```python
from build123d import *

# Parameters (mm, degrees)
BOSS_EXTRUDE1_DEPTH = 3.81


with BuildPart() as part:
    # Sketch1 → Boss-Extrude1 (new body)
    with BuildSketch(Plane.XY):
        with BuildLine():
            Line((-43.434, -9.779), (-43.434, -14.224))
            Line((-43.434, -14.224), (-34.544, -14.224))
            Line((-34.544, -14.224), (-34.544, -9.779))
            Line((-34.544, -9.779), (-34.544, -8.876475723))
            ThreePointArc((-34.544, -8.876475723), (-34.231125677, -8.041724001), (-33.446660728, -7.618267365))
            Line((-33.446660728, -7.618267365), (-11.222947321, -4.568563784))
            ThreePointArc((-11.222947321, -4.568563784), (0, -3.802107076), (11.222947321, -4.568563784))
            Line((11.222947321, -4.568563784), (33.446660728, -7.618267365))
            ThreePointArc((33.446660728, -7.618267365), (34.231125677, -8.041724001), (34.544, -8.876475723))
            Line((34.544, -8.876475723), (34.544, -9.779))
            Line((34.544, -9.779), (34.544, -14.224))
            Line((34.544, -14.224), (43.434, -14.224))
            Line((43.434, -14.224), (43.434, -9.779))
            Line((43.434, -9.779), (43.434, -6.250721328))
            ThreePointArc((43.434, -6.250721328), (43.288497568, -5.660462724), (42.885330364, -5.205454612))
            ThreePointArc((42.885330364, -5.205454612), (42.48216316, -4.7504465), (42.336660728, -4.160187897))
            Line((42.336660728, -4.160187897), (42.336660728, 4.160187897))
            ThreePointArc((42.336660728, 4.160187897), (42.48216316, 4.7504465), (42.885330364, 5.205454612))
            ThreePointArc((42.885330364, 5.205454612), (43.288497568, 5.660462724), (43.434, 6.250721328))
            Line((43.434, 6.250721328), (43.434, 9.779))
            Line((43.434, 9.779), (43.434, 14.224))
            Line((43.434, 14.224), (34.544, 14.224))
            Line((34.544, 14.224), (34.544, 9.779))
            Line((34.544, 9.779), (34.544, 8.876475723))
            ThreePointArc((34.544, 8.876475723), (34.231125677, 8.041724001), (33.446660728, 7.618267365))
            Line((33.446660728, 7.618267365), (11.222947321, 4.568563784))
            ThreePointArc((11.222947321, 4.568563784), (0, 3.802107076), (-11.222947321, 4.568563784))
            Line((-11.222947321, 4.568563784), (-33.446660728, 7.618267365))
            ThreePointArc((-33.446660728, 7.618267365), (-34.231125677, 8.041724001), (-34.544, 8.876475723))
            Line((-34.544, 8.876475723), (-34.544, 9.779))
            Line((-34.544, 9.779), (-34.544, 14.224))
            Line((-34.544, 14.224), (-43.434, 14.224))
            Line((-43.434, 14.224), (-43.434, 9.779))
            Line((-43.434, 9.779), (-43.434, 6.250721328))
            ThreePointArc((-43.434, 6.250721328), (-43.288497568, 5.660462724), (-42.885330364, 5.205454612))
            ThreePointArc((-42.885330364, 5.205454612), (-42.48216316, 4.7504465), (-42.336660728, 4.160187897))
            Line((-42.336660728, 4.160187897), (-42.336660728, -4.160187897))
            ThreePointArc((-42.336660728, -4.160187897), (-42.48216316, -4.7504465), (-42.885330364, -5.205454612))
            ThreePointArc((-42.885330364, -5.205454612), (-43.288497568, -5.660462724), (-43.434, -6.250721328))
            Line((-43.434, -6.250721328), (-43.434, -9.779))
        make_face()
        with BuildLine():
            Line((-33.101339272, -3.725173331), (-15.12414212, -1.258208358))
            ThreePointArc((-15.12414212, -1.258208358), (-14.026802848, 0), (-15.12414212, 1.258208358))
            Line((-15.12414212, 1.258208358), (-33.101339272, 3.725173331))
            ThreePointArc((-33.101339272, 3.725173331), (-34.108751722, 3.42409065), (-34.544, 2.466964972))
            Line((-34.544, 2.466964972), (-34.544, -2.466964972))
            ThreePointArc((-34.544, -2.466964972), (-34.108751722, -3.42409065), (-33.101339272, -3.725173331))
        make_face(mode=Mode.SUBTRACT)
        with BuildLine():
            Line((34.544, -2.466964972), (34.544, 2.466964972))
            ThreePointArc((34.544, 2.466964972), (34.108751722, 3.42409065), (33.101339272, 3.725173331))
            Line((33.101339272, 3.725173331), (15.12414212, 1.258208358))
            ThreePointArc((15.12414212, 1.258208358), (14.026802848, 0), (15.12414212, -1.258208358))
            Line((15.12414212, -1.258208358), (33.101339272, -3.725173331))
            ThreePointArc((33.101339272, -3.725173331), (34.108751722, -3.42409065), (34.544, -2.466964972))
        make_face(mode=Mode.SUBTRACT)
    extrude(amount=BOSS_EXTRUDE1_DEPTH)


solid = part.part
```
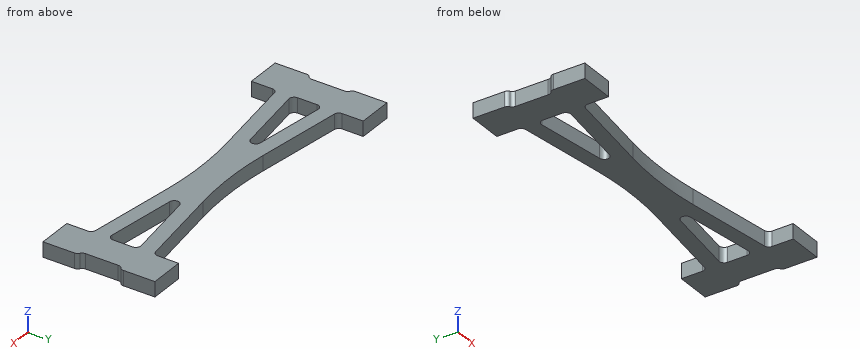
Geometry: final body of the model. Coordinates: model frame, mm. Round coordinates to 2 decimals unless told otherwise and drop trailing zeros. Write each loop counter-clockwise with the first axis right and the second up, starting at its lowest first coordinate (ties: lowest second). Pieces come first, ordered by that corner, then holes. Notation, with made-up numbers: (9.5, 14) -> (61.5, 14) arc R37 ccw to (61.5, 53) -> close; hole circle Ø8 at (-7, 0). An arc over 180 degrees is marked (long way). Use CSV: the item, a comma, the result in double quotes. Start each with the question number.
Q1. Section A-A (y = -10.5). Return loops of the section in (x, z), plus the area to 3 significant figures.
Q2. Section C-C (y = 0.25). Return loops of the section in (x, z), plus the area to 3 significant figures.
Q3. First-contact query: pin 1 Ø1.9 at (y, z) = (0, 1.5) entering from +X; pin 2 Ø1.5 at (x, z) = (-29, 2.5) entering from +Y; pin 3 Ø1.5 at (y, z) = (-0.5, 3.5) entering from -X. Flat tips, straight axial feed; report the tip coordinate or a pass-through.
Q4. Section B-B (x = -16.5). Return loops of the section in (y, z), plus the area to 3 significant figures.
Q5. Line query: L1, parallel to X at y = -13, z = 2.25; L2, parallel to X at y = -0.25, z = 3.45; L3, parallel to Y at x = -16.5, z = 3.65. Output: solid intervals per line, ascending.
Q6. Section D-D (z = 2.2). Give the number of separate pieces and of enclosed holes in the cut face, plus the area to 3 significant figures.
Result sheet:
1,outline,"(-43.43, 0) -> (-34.54, 0) -> (-34.54, 3.81) -> (-43.43, 3.81) -> close; (34.54, 0) -> (43.43, 0) -> (43.43, 3.81) -> (34.54, 3.81) -> close"
1,area,"67.7 mm²"
2,outline,"(-42.34, 0) -> (-34.54, 0) -> (-34.54, 3.81) -> (-42.34, 3.81) -> close; (-14.05, 0) -> (14.05, 0) -> (14.05, 3.81) -> (-14.05, 3.81) -> close; (34.54, 0) -> (42.34, 0) -> (42.34, 3.81) -> (34.54, 3.81) -> close"
2,area,"166 mm²"
3,pin 1,"x = 42.34"
3,pin 2,"y = 7.11"
3,pin 3,"x = -42.34"
4,outline,"(-5.29, 0) -> (-1.45, 0) -> (-1.45, 3.81) -> (-5.29, 3.81) -> close; (1.45, 0) -> (5.29, 0) -> (5.29, 3.81) -> (1.45, 3.81) -> close"
4,area,"29.3 mm²"
5,L1,"-43.43 to -34.54, 34.54 to 43.43"
5,L2,"-42.34 to -34.54, -14.05 to 14.05, 34.54 to 42.34"
5,L3,"-5.29 to -1.45, 1.45 to 5.29"
6,separate pieces,"1"
6,enclosed holes,"2"
6,area,"1,040 mm²"
